Input: part model. Units: mm. Frame: model coordinates. A direction names the side the tool comes from. Round coordinates to 2 decimals unless told otherwise and drop trailing zeros. Loops run counter-clockwise (first coordinate to the right, second up) from the corner with the lowest first, then second, coordinate; pieces in that order, holes last.
(1) Cut plane B-B, the plane y = 42. Output: boundary loops of the cut face in (x, z).
(2) Cut plane C-C, the plane x = -40. Output: boundary loops of the cut face in (y, z), and give its area (3 significant figures).
(3) Cut plane A-A, the plane z = -3.5. Output: boundary loops of the cut face in (x, y), and give its area (3 significant figures).
(4) First-contact query: pin 1 Ø0.8 at (x, y) = (0, -28) entering from +Z; pin 2 Ø7.5 at (y, z) = (4.5, -3.5) entering from -X; pin 3 Ø3 at (y, z) = (4, -7) entering from +X. Flat tips, straight axial feed; report the tip coordinate or a pass-through.
(5) Draft query along Y for faces 6 (the face through (0, 6, -9.5)), 7 (the face through (-32.12, 30.02, -28.49)), 8 (the face through (-31, 38, -28)). Return one class per face: released by +Y, released by -Y, zero draft, split by the parting line, or undercut.
(6) Cut plane D-D, the plane z = -16.25. Output: boundary loops of the cut face in (x, y), and give its area (3 significant figures).
(7) Line query: line 1 (X direction, y = -7.5, z = -9); line 2 (Z direction, x = -6, y = -22); line 3 (Z direction, x = -17.5, y = 43). Output: solid intervals per line, ascending.
(8) Access query for faces 1 (the face through (0, -31, -14)), 2 (the face through (2.55, 42.73, -18.62)), 3 (the face through (8.822, 37.3, -28.493)), 4 (the face through (9.5, -1, -5)), 5 (the face through (-31, 38, -29)). Directions: +Z, -Z, +X, -X, +Y, -Y. A direction counts if a zero-diameter tool reaches every point of the face in a straight line with its end or side. Return the directions, or none.
from build123d import *

# Parameters (mm, degrees)
EXTRUDE_1_DEPTH     = 9.5
SKETCH_2_W          = 18
SKETCH_2_H          = 11
EXTRUDE_2_DEPTH     = 4.5
EXTRUDE_2_TAPER     = 15
SKETCH_3_R          = 5
CUT_EXTRUDE_1_DEPTH = 5
SKETCH_4_R          = 4.9
EXTRUDE_3_DEPTH     = 5
SKETCH_5_W          = 0.978234864
SKETCH_5_H          = 6.839106706
CUT_EXTRUDE_2_DEPTH = 0.1
SKETCH_7_R          = 5.9
EXTRUDE_4_DEPTH     = 18.5
EXTRUDE_5_DEPTH     = 1


with BuildPart() as part:
    # 草圖1 → 伸長1 (new body)
    with BuildSketch(Plane.XY):
        with BuildLine():
            Line((-9.5, 36), (-9.5, -37))
            Line((-9.5, -37), (9.5, -37))
            Line((9.5, -37), (9.5, 36))
            ThreePointArc((9.5, 36), (0, 47.117692031), (-9.5, 36))
        make_face()
    extrude(amount=-EXTRUDE_1_DEPTH)

    # 草圖2 → 伸長2 (add)
    with BuildSketch(Plane(origin=(0, 0, -9.5), x_dir=(-1, 0, 0), z_dir=(0, 0, -1))):
        with Locations((0, -31)):
            Rectangle(SKETCH_2_W, SKETCH_2_H)
    extrude(amount=EXTRUDE_2_DEPTH, taper=EXTRUDE_2_TAPER)

    # 草圖3 → 除料-伸長1 (cut)
    with BuildSketch(Plane.XY):
        with Locations((0, -28.150570544)):
            Circle(SKETCH_3_R)
    extrude(amount=-CUT_EXTRUDE_1_DEPTH, mode=Mode.SUBTRACT)

    # 草圖4 → 伸長3 (add)
    with BuildSketch(Plane.XY.offset(-5)):
        with Locations((0, -28.150570544)):
            Circle(SKETCH_4_R)
    extrude(amount=EXTRUDE_3_DEPTH)

    # 草圖5 → 除料-伸長2 (cut)
    with BuildSketch(Plane.XY):
        with Locations((0, -28.150570544)):
            Rectangle(SKETCH_5_W, SKETCH_5_H)
    extrude(amount=-CUT_EXTRUDE_2_DEPTH, mode=Mode.SUBTRACT)

    # 草圖7 → 伸長4 (add)
    with BuildSketch(Plane(origin=(0, 0, -9.5), x_dir=(-1, 0, 0), z_dir=(0, 0, -1))):
        with Locations(Location((0.17562961, 37.497796385, 0), (0, 0, 180))):
            Circle(SKETCH_7_R)
    extrude(amount=EXTRUDE_4_DEPTH)

    # 草圖8 → 伸長5 (add)
    with BuildSketch(Plane(origin=(0, 0, -28), x_dir=(-1, 0, 0), z_dir=(0, 0, -1))):
        with BuildLine():
            Line((0.17562961, 46.497796385), (63.17562961, 43.497796385))
            ThreePointArc((63.17562961, 43.497796385), (69.17562961, 37.497796385), (63.17562961, 31.497796385))
            Line((63.17562961, 31.497796385), (0.17562961, 28.497796385))
            ThreePointArc((0.17562961, 28.497796385), (-8.82437039, 37.497796385), (0.17562961, 46.497796385))
        make_face()
    extrude(amount=EXTRUDE_5_DEPTH)


solid = part.part
Reported:
1. outline: (-67.14, -29) - (7.62, -29) - (7.62, -28) - (3.64, -28) - (3.64, -9.5) - (8.5, -9.5) - (8.5, 0) - (-8.5, 0) - (-8.5, -9.5) - (-3.99, -9.5) - (-3.99, -28) - (-67.14, -28) - close
2. outline: (30.39, -29) - (44.6, -29) - (44.6, -28) - (30.39, -28) - close
2. area: 14.2 mm2
3. outline: (-9.5, -37) - (9.5, -37) - (9.5, 36) arc R9.62 ccw (long way) to (-9.5, 36) - close; circle Ø9.8 at (0, -28.15); hole circle Ø10 at (0, -28.15)
3. area: 1,560 mm2
4. pin 1: stops at z = -0.1
4. pin 2: stops at x = -9.5
4. pin 3: stops at x = 9.5
5. face 6: undercut
5. face 7: released by -Y
5. face 8: zero draft
6. outline: circle Ø11.8 at (-0.18, 37.5)
6. area: 109 mm2
7. line 1: x = -9.5 to 9.5
7. line 2: z = -9.5 to 0
7. line 3: z = -29 to -28
8. face 1: -Z, +X, -X, -Y
8. face 2: none
8. face 3: -Z, +X
8. face 4: +Z, -Z, +X, -Y
8. face 5: -Z, +X, -X, +Y, -Y
